Read the model definition and answer for the solid it produces. Units are mm, in the model's axes. Face numbers are marked on the shaded views. A direction names the side the tool comes from. Round coordinates to 2 decimals unless told otherwise and drop trailing zeros. Order: outer loops, then holes, each group sorted by start corner. A loop starts at its lowest first (then second) coordinate and runs counter-clockwise, first axis right, second up. Notation, with made-up numbers: (28.25, -27) -> (84.25, -27) arc R19 cw to (84.25, 6) -> close; hole circle Ø5 at (25.25, -31.75). An arc over 180 degrees is marked (long way). Use a Markdown table: item, result. Add a question column.
1. Given pin 1 (1 mm diameter, centred on x = 8, z = -0.5, fed in from -Y) (3 decimals); pin 2 (3.5 mm diameter, centred on x = -2, z = 1, fed in from -Y) (3 decimals); pin 3 (2 mm diameter, centred on x = 12, z = -1.5, fed in from +Y), each flat-ended and moving along its own axis, determine where each tip first touches the part or whether it passes through.
2. Section C-C, the plane x = 11.5 is taken. Give the vertices of the cut face in (y, z) (3 decimals).
3. For the marked faces 4, 5 and 6, determine the directions among +Z, -Z, +X, -X, +Y, -Y from which every point of the face is accessible in a straight line to the end or side of a thin tool.
4. Section D-D, the plane y = 1.5 is taken. Give the vertices of the cut face in (x, z) (3 decimals), then the cut area to 3 significant figures.
5. Consider L1, parallel to X at y = -1.25, z = 0 (3 decimals); L2, parallel to X at y = 9.5, z = 0 (3 decimals); L3, parallel to X at y = 3, z = 0 (3 decimals). Determine where each line is inside the solid, lowest interval first. Write a range as [from, to].
6. Section B-B, the plane z = 0 is taken. Give the vertices of the cut face in (x, y) (3 decimals).
7. The mould has two halves that part along Z. Classify the marked faces 1, 2 and 3: +Z half, -Z half, draft (parallel to the pull), parting line (faces both ways), or undercut.
8. Section A-A, the plane y = -3.25 is taken. Give the vertices of the cut face in (x, z) (3 decimals).
Autodesk Inventor part; units mm, degrees
ref_plane "YZ Plane" through (0, 0, 0) normal (1, 0, 0) x (0, 1, 0)
ref_plane "XZ Plane" through (0, 0, 0) normal (0, 1, 0) x (-1, 0, 0)
ref_plane "XY Plane" through (0, 0, 0) normal (0, 0, 1) x (1, 0, 0)
sketch "Mount Shape Sketch" plane through (0, 0, 0) normal (0, 0, 1) x (1, 0, 0)
  circle A0 centre (0, 0) radius 8.115
  line L0 (-5.4362, 6.025) -> (5.4362, 6.025)
  line L1 (-5.4362, -6.025) -> (5.4362, -6.025)
  line L2 (-8.115, 0) -> (-8.115, -5.525)
  line L3 (8.115, 0) -> (8.115, -5.525)
  line L4 (8.115, -5.525) -> (15, -5.525)
  line L5 (15, -5.525) -> (15, 12.9873)
  line L6 (15, 12.9873) -> (-15, 12.9873)
  line L7 (-15, 12.9873) -> (-15, -5.525)
  line L8 (-15, -5.525) -> (-8.115, -5.525)
  line L9 (0, 17.2077) -> (0, -12.3355) construction
  dimension "d0" = 16.23
  dimension "d1" = 12.05
  dimension "d3" = 30
  dimension "d15" = 12.9873
  dimension "d18" = 0.5
extrude "Mount Shape" add sketch "Mount Shape Sketch" along normal mid plane 15 contours A0 L2 L8 L7 L6 L5 L4 L3 | L0 A0
sketch "Sketch2" plane through (-15, 12.9873, 7.5) normal (0, 1, 0) x (1, 0, 0)
  circle A0 centre (3.585, 7.5) radius 1.75
  line L0 (20.4362, 15) -> (9.5638, 15) construction
  line L1 (15, 15) -> (15, 0) construction
  line L2 (30, 0) -> (0, 0) construction
  line L3 (15, 7.5) -> (3.585, 7.5) construction
  circle A1 centre (26.415, 7.5) radius 1.75
  dimension "d6" = 3.5
  dimension "d7" = 11.415
  dimension "d14" = 22.83
extrude "Screw Shaft Holes" cut sketch "Sketch2" against normal through all
sketch "Sketch3" plane through (-15, 12.9873, 7.5) normal (0, 1, 0) x (1, 0, 0)
  circle A0 centre (3.585, 7.5) radius 1.75
  circle A1 centre (3.585, 7.5) radius 3.25
  circle A2 centre (26.415, 7.5) radius 3.25
  circle A3 centre (26.415, 7.5) radius 1.75
  point P0 (15, 7.5)
  dimension "d10" = 6.5
extrude "Screw Head Holes" cut sketch "Sketch3" against normal blind 6.8 contours A0 | A1 | A2 | A3
fillet "Outer Fillet" radius 1 4 edges at (15, 3.7311, -7.5) (15, 3.7311, 7.5) (-15, 3.7311, 7.5) (-15, 3.7311, -7.5)
properties part number "Large Drive Motors Mount Cap"
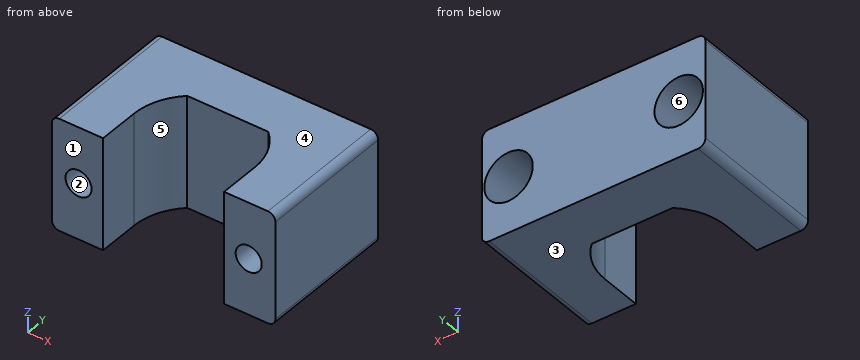
Verdict:
| question | item | result |
|---|---|---|
| 1 | pin 1 | stops at y = -5.525 |
| 1 | pin 2 | stops at y = 6.025 |
| 1 | pin 3 | stops at y = 6.19 |
| 2 | outline | (-5.525, -7.5) -> (12.987, -7.5) -> (12.987, -3.249) -> (6.187, -3.249) -> (6.187, -1.748) -> (-5.525, -1.748) -> close; (-5.525, 1.748) -> (6.187, 1.748) -> (6.187, 3.249) -> (12.987, 3.249) -> (12.987, 7.5) -> (-5.525, 7.5) -> close |
| 3 | face 4 | +Z, +X, -X, +Y, -Y |
| 3 | face 5 | +Z, -Z, -Y |
| 3 | face 6 | +Y |
| 4 | outline | (-15, -6.5) arc R1 ccw to (-14, -7.5) -> (-7.975, -7.5) -> (-7.975, 7.5) -> (-14, 7.5) arc R1 ccw to (-15, 6.5) -> close; (7.975, -7.5) -> (14, -7.5) arc R1 ccw to (15, -6.5) -> (15, 6.5) arc R1 ccw to (14, 7.5) -> (7.975, 7.5) -> close; hole circle Ø3.5 at (-11.415, 0); hole circle Ø3.5 at (11.415, 0) |
| 4 | area | 191 mm2 |
| 5 | L1 | x = [-15, -13.165], [-9.665, -8.115], [8.115, 9.665], [13.165, 15] |
| 5 | L2 | x = [-15, -14.665], [-8.165, 8.165], [14.665, 15] |
| 5 | L3 | x = [-15, -13.165], [-9.665, -7.54], [7.54, 9.665], [13.165, 15] |
| 6 | outline | (-15, -5.525) -> (-13.165, -5.525) -> (-13.165, 6.187) -> (-14.665, 6.187) -> (-14.665, 12.987) -> (-15, 12.987) -> close; (-9.665, -5.525) -> (-8.115, -5.525) -> (-8.115, 0) arc R8.115 cw to (-5.436, 6.025) -> (5.436, 6.025) arc R8.115 cw to (8.115, 0) -> (8.115, -5.525) -> (9.665, -5.525) -> (9.665, 6.187) -> (8.165, 6.187) -> (8.165, 12.987) -> (-8.165, 12.987) -> (-8.165, 6.187) -> (-9.665, 6.187) -> close; (13.165, -5.525) -> (15, -5.525) -> (15, 12.987) -> (14.665, 12.987) -> (14.665, 6.187) -> (13.165, 6.187) -> close |
| 7 | face 1 | draft |
| 7 | face 2 | undercut |
| 7 | face 3 | -Z half |
| 8 | outline | (-15, -6.5) arc R1 ccw to (-14, -7.5) -> (-8.115, -7.5) -> (-8.115, 7.5) -> (-14, 7.5) arc R1 ccw to (-15, 6.5) -> close; (8.115, -7.5) -> (14, -7.5) arc R1 ccw to (15, -6.5) -> (15, 6.5) arc R1 ccw to (14, 7.5) -> (8.115, 7.5) -> close; hole circle Ø3.5 at (-11.415, 0); hole circle Ø3.5 at (11.415, 0) |
